```python
from build123d import *

# Parameters (mm, degrees)
F0_W     = 60.5
F0_H     = 60.5
F1_DEPTH = 5
F2_DEPTH = 6.5


with BuildPart() as f1:
    # F0 (on Top) → F1 (new body)
    with BuildSketch(Plane.XY):
        Polygon((3.5355339059, -12.5), (3.5355339059, 12.5), (3.5355339059, 33.7855339059), (-64.0355339059, 33.7855339059), (-64.0355339059, -33.7855339059), (3.5355339059, -33.7855339059), align=None)
        with Locations((-30.25, 0)):
            Rectangle(F0_W, F0_H, mode=Mode.SUBTRACT)
        with Locations((-30.25, 0)):
            Rectangle(F0_W, F0_H)
    extrude(amount=F1_DEPTH)

    # F0 (on Top) → F2 (join)
    with BuildSketch(Plane.XY):
        Polygon((3.5355339059, -12.5), (3.5355339059, 12.5), (3.5355339059, 33.7855339059), (-64.0355339059, 33.7855339059), (-64.0355339059, -33.7855339059), (3.5355339059, -33.7855339059), align=None)
        with Locations((-30.25, 0)):
            Rectangle(F0_W, F0_H, mode=Mode.SUBTRACT)
    extrude(amount=F2_DEPTH)


solid = f1.part
```
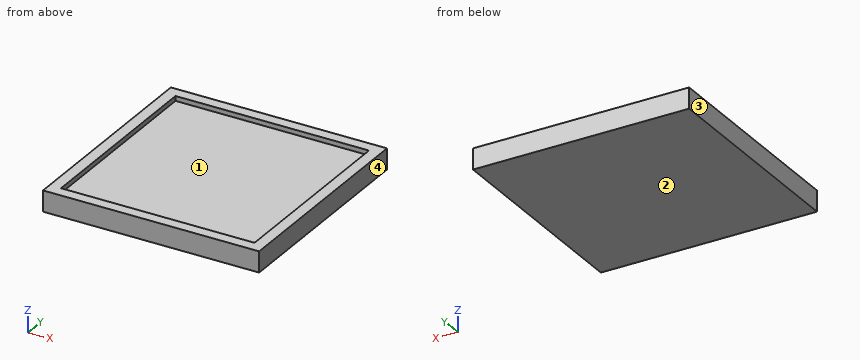
Check sheet for the modelled part. Datum: model origin and axes. Units: mm. Face numbers are marked on the shaded views. Give positions to 0.01 mm unless a question says otherwise; leave off trailing zeros. Write each loop counter-clockwise with the first axis right and the second up, starting at its lowest first coordinate (ties: lowest second). Pieces come first, ordered by that corner, then holes. Notation, with made-up numbers: (19.5, 7) - (28.5, 7) arc R31 ccw to (28.5, 46) - close; hole circle Ø2 at (-2.75, 3.5). An arc over 180 degrees is marked (long way). Answer as a JSON object with one key per item and string values. Group by question number.
1) Release check for a two-part mould opening along X. For the marked faces 1, 2, 3 and 4 record: pulls with the +X half, pulls with the -X half, needs draft (parallel to the pull), parting line crosses it, or undercut.
2) Depth check by flat-ended pin: P1, Ø1.5, axis at x = -39.5, y = -15, coming from the +Z side. Enter the tip coordinate at first touch or a pass-through.
3) Sectioned sample at B-B (y = 8.5). Record the cut outline in (x, z), then the cut area to 3 significant figures.
4) Sectioned sample at A-A (x = -13). Record the cut outline in (y, z), then the cut area to 3 significant figures.
5) Thickness scan on probe 1 along X at (y, z) = (0, 6.25); probe 2 along Y at (x, z) = (-12, 6.25); probe 3 along Z at (x, y) = (-20, -17). Record the ranges inside material, lowest first. Write a range as from..to.
Geometry results:
{
 "1": {"face 1": "undercut", "face 2": "needs draft", "face 3": "pulls with the -X half", "face 4": "pulls with the +X half"},
 "2": {"P1": "stops at z = 5"},
 "3": {"outline": "(-64.04, 0) - (3.54, 0) - (3.54, 6.5) - (0, 6.5) - (0, 5) - (-60.5, 5) - (-60.5, 6.5) - (-64.04, 6.5) - close", "area": "348 mm^2"},
 "4": {"outline": "(-33.79, 0) - (33.79, 0) - (33.79, 6.5) - (30.25, 6.5) - (30.25, 5) - (-30.25, 5) - (-30.25, 6.5) - (-33.79, 6.5) - close", "area": "348 mm^2"},
 "5": {"probe 1": "x = -64.04..-60.5, 0..3.54", "probe 2": "y = -33.79..-30.25, 30.25..33.79", "probe 3": "z = 0..5"}
}
